```python
from build123d import *

# Parameters (mm, degrees)
F2_R     = 22.5
F2_R_2   = 12.5
F3_DEPTH = 12.5
F4_COUNT = 4
F4_ANGLE = 270


with BuildPart() as f1:
    # F0 (on Front) → F1 (revolve)
    with BuildSketch(Plane.XZ):
        with BuildLine():
            ThreePointArc((0, -72.5), (51.265241636, -51.265241636), (72.5, 0))
            ThreePointArc((72.5, 0), (65.2241802056, 15.4303349962), (48.6904761905, 19.6338363125))
            ThreePointArc((48.6904761905, 19.6338363125), (32.5, 0), (48.6904761905, -19.6338363125))
            ThreePointArc((48.6904761905, -19.6338363125), (29.3723815309, -43.5145171546), (0, -52.5))
            Line((0, -52.5), (0, -72.5))
        make_face()
    revolve(axis=Axis((0, 0, 0), (0, 0, -1)))

    # F2 (on Right) → F3 (join, symmetric)
    with BuildSketch(Plane.YZ):
        with Locations((75, 0)):
            Circle(F2_R)
        with Locations((75, 0)):
            Circle(F2_R_2, mode=Mode.SUBTRACT)
    extrude(amount=F3_DEPTH, both=True)

    # F4: F1 ×4 about axis
    f4_axis = Axis((0, 0, 0), (0, 0, -1))


with BuildPart() as f1_1:
    add(f1.part)
    for i in range(1, F4_COUNT):
        add(f1.part.rotate(f4_axis, i * F4_ANGLE / (F4_COUNT - 1)))


solid = f1_1.part
```
Build history of the part. All positions in model axes, mm. Coordinates: 2 decimals unless noted, no trailing zeros. Write each loop counter-clockwise with the first axis right and the second up, starting at its lowest first coordinate (ties: lowest second). Pieces come first, ordered by that corner, then holes.
1. Band-saw the part on D-D, the plane y = 8. Give the number of separate pieces and of enclosed holes in the cut face, and give its area (3 significant figures).
Answer block:
separate pieces: 1
enclosed holes: 2
area: 7,190 mm2
2. Band-saw the part on A-A, the plane x = 75. Give the cut face in (y, z).
Answer block:
outline: (-12.5, -22.5) - (12.5, -22.5) - (12.5, -12.5) - (-12.5, -12.5) - close; (-12.5, 12.5) - (12.5, 12.5) - (12.5, 22.5) - (-12.5, 22.5) - close
3. Drop flat-ended pins along their axis: pin 1 (8 mm diameter, centred on y = 6.5, z = -59.5, fed in from +X); pin 2 (22.5 mm diameter, centred on y = -75, z = 0, fed in from -X); pin 3 (11 mm diameter, centred on x = 82, z = -6.5, fed in from -Y). Give the stop position or say it passes through.
Answer block:
pin 1: stops at x = 46.22
pin 2: stops at x = -34.53
pin 3: stops at y = -12.5
4. Band-saw the part on C-C, the plane z = -8. Give the cut face in (x, y).
Answer block:
outline: (-96.03, -12.5) - (-84.6, -12.5) - (-84.6, 12.5) - (-96.03, 12.5) - close; circle Ø144.11 at (0, 0); (-12.5, -96.03) - (12.5, -96.03) - (12.5, -84.6) - (-12.5, -84.6) - close; (-12.5, 84.6) - (12.5, 84.6) - (12.5, 96.03) - (-12.5, 96.03) - close; (84.6, -12.5) - (96.03, -12.5) - (96.03, 12.5) - (84.6, 12.5) - close; hole circle Ø68.34 at (0, 0)
5. Pull direction Y, two halves, no side cores. Call faces 1 (the flat face through (-87, 12.5, 5)), 2 (the cylindrical face through (0.175, -87.472, 0.831)), 3 (the flat face through (12.5, -87, 5)): released by +Y, released by -Y, zero draft, split by the parting line, or undercut.
Answer block:
face 1: released by +Y
face 2: undercut
face 3: zero draft
6. Drill centre lines: probe 1 along Z at (x, y) = (75, 0); probe 2 along X at (y, z) = (6, 0); probe 3 along X at (y, z) = (-1.5, 0). Where is each one in solid material? Low to high.
Answer block:
probe 1: z = -22.5 to -12.5, 12.5 to 22.5
probe 2: x = -97.5 to -87.5, -72.25 to -31.94, 31.94 to 72.25, 87.5 to 97.5
probe 3: x = -97.5 to -87.5, -72.48 to -32.47, 32.47 to 72.48, 87.5 to 97.5
